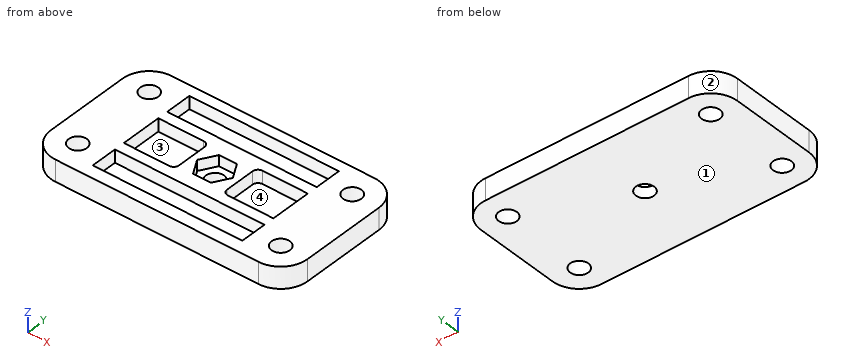
```python
from build123d import *

# Parameters (mm, degrees)
SKETCH1_R           = 1.7
BOSS_EXTRUDE1_DEPTH = 4
CUT_EXTRUDE1_DEPTH  = 2
SKETCH3_W           = 28
SKETCH3_H           = 4.960661027
SKETCH3_W_2         = 9.5
SKETCH3_H_2         = 7.70604726
SKETCH3_H_3         = 4.960661028
CUT_EXTRUDE2_DEPTH  = 2.4
FILLET1_R           = 1


with BuildPart() as part:
    # Sketch1 → Boss-Extrude1 (new body)
    with BuildSketch(Plane.XY):
        with BuildLine():
            Line((-19, -13), (19, -13))
            ThreePointArc((19, -13), (22.535533906, -11.535533906), (24, -8))
            Line((24, -8), (24, 8))
            ThreePointArc((24, 8), (22.535533906, 11.535533906), (19, 13))
            Line((19, 13), (-19, 13))
            ThreePointArc((-19, 13), (-22.535533906, 11.535533906), (-24, 8))
            Line((-24, 8), (-24, -8))
            ThreePointArc((-24, -8), (-22.535533906, -11.535533906), (-19, -13))
        make_face()
        Circle(SKETCH1_R, mode=Mode.SUBTRACT)
        with Locations((19, 8)):
            Circle(SKETCH1_R, mode=Mode.SUBTRACT)
        with Locations((19, -8)):
            Circle(SKETCH1_R, mode=Mode.SUBTRACT)
        with Locations((-19, -8)):
            Circle(SKETCH1_R, mode=Mode.SUBTRACT)
        with Locations((-19, 8)):
            Circle(SKETCH1_R, mode=Mode.SUBTRACT)
    extrude(amount=BOSS_EXTRUDE1_DEPTH)

    # Sketch2 → Cut-Extrude1 (cut)
    with BuildSketch(Plane.XY.offset(4)):
        Polygon((3.348631561, 0), (1.674315781, 2.9), (-1.674315781, 2.9), (-3.348631561, 0), (-1.674315781, -2.9), (1.674315781, -2.9), align=None)
    extrude(amount=-CUT_EXTRUDE1_DEPTH, mode=Mode.SUBTRACT)

    # Sketch3 → Cut-Extrude2 (cut)
    with BuildSketch(Plane.XY.offset(4)):
        with Locations((0, 8.519669486)):
            Rectangle(SKETCH3_W, SKETCH3_H)
        with Locations((-9.25, 0.186315343)):
            Rectangle(SKETCH3_W_2, SKETCH3_H_2)
        with Locations((9.25, 0.186315343)):
            Rectangle(SKETCH3_W_2, SKETCH3_H_2)
        with Locations((0, -8.147038801)):
            Rectangle(SKETCH3_W, SKETCH3_H_3)
    extrude(amount=-CUT_EXTRUDE2_DEPTH, mode=Mode.SUBTRACT)

    # Fillet1
    fillet1_edges = [part.edges().sort_by_distance(p)[0] for p in [
        (-4.5, 4.039338973, 2.8),
        (-4.5, -3.666708287, 2.8),
        (4.5, -3.666708287, 2.8),
        (4.5, 4.039338973, 2.8),
    ]]
    fillet(fillet1_edges, radius=FILLET1_R)


solid = part.part
```
The listing builds one solid part. Answer for the finished solid, in the listing's coordinates (mm). Face numbers are marked on the shaded views. Give positions to 0.01 mm unless a question says otherwise; leave off trailing zeros. Loops run counter-clockwise (first coordinate to the right, second up) from the corner with the lowest first, then second, coordinate; pieces in that order, holes last. Notation, with made-up numbers: (-13, 15.5) - (1, 15.5) arc R15 cw to (1, 34.5) - close; hole circle Ø10 at (23.5, 38.25). An arc over 180 degrees is marked (long way). Answer as CSV lines item,"result". Start each with the question number.
Item 1: A cutting plane is placed at B-B on z = 0.55. Determine the outline of the cut face in (x, y).
Item 2: Each of these flat-tipped pins is pushed along its axis until it touches: pin 1 (4 mm diameter, centred on x = 1, y = -9.5, fed in from +Z); pin 2 (1.5 mm diameter, centred on x = -4, y = -7.5, fed in from +Z). Where does it stop, or does it pass through?
Item 3: A cutting plane is placed at D-D on y = 7.5. Determine the outline of the cut face in (x, z), then the cut area to 3 significant figures.
Item 4: Find the intervals of material crossed by line 1 (Y direction, x = 0.5, z = 2.7); line 2 (Y direction, x = 19, z = 2.55); line 3 (Y direction, x = 10, z = 3.15), in increasing order. Write a range as from..to.
Item 5: A cutting plane is placed at A-A on x = 0. Determine the outline of the cut face in (y, z), then the cut area to 3 significant figures.
Item 6: The mould has two halves that part along X. Classify the marked faces 1, 2, 3 and 4: +X half, -X half, draft (parallel to the pull), parting line (faces both ways), or undercut.
Item 7: A cutting plane is placed at C-C on x = -6.5. Determine the outline of the cut face in (y, z).
Found:
1,outline,"(-24, -8) arc R5 ccw to (-19, -13) - (19, -13) arc R5 ccw to (24, -8) - (24, 8) arc R5 ccw to (19, 13) - (-19, 13) arc R5 ccw to (-24, 8) - close; hole circle Ø3.4 at (-19, -8); hole circle Ø3.4 at (-19, 8); hole circle Ø3.4 at (0, 0); hole circle Ø3.4 at (19, -8); hole circle Ø3.4 at (19, 8)"
2,pin 1,"stops at z = 4"
2,pin 2,"stops at z = 1.6"
3,outline,"(-24, 0) - (-20.62, 0) - (-20.62, 4) - (-24, 4) - close; (-17.38, 0) - (17.38, 0) - (17.38, 4) - (14, 4) - (14, 1.6) - (-14, 1.6) - (-14, 4) - (-17.38, 4) - close; (20.62, 0) - (24, 0) - (24, 4) - (20.62, 4) - close"
3,area,"98.8 mm^2"
4,line 1,"y = -13..-10.63, -5.67..-2.9, 2.9..6.04, 11..13"
4,line 2,"y = -13..-9.7, -6.3..6.3, 9.7..13"
4,line 3,"y = -13..-10.63, -5.67..-3.67, 4.04..6.04, 11..13"
5,outline,"(-13, 0) - (-1.7, 0) - (-1.7, 2) - (-2.9, 2) - (-2.9, 4) - (-5.67, 4) - (-5.67, 1.6) - (-10.63, 1.6) - (-10.63, 4) - (-13, 4) - close; (1.7, 0) - (13, 0) - (13, 4) - (11, 4) - (11, 1.6) - (6.04, 1.6) - (6.04, 4) - (2.9, 4) - (2.9, 2) - (1.7, 2) - close"
5,area,"61.8 mm^2"
6,face 1,"draft"
6,face 2,"-X half"
6,face 3,"undercut"
6,face 4,"undercut"
7,outline,"(-13, 0) - (13, 0) - (13, 4) - (11, 4) - (11, 1.6) - (6.04, 1.6) - (6.04, 4) - (4.04, 4) - (4.04, 1.6) - (-3.67, 1.6) - (-3.67, 4) - (-5.67, 4) - (-5.67, 1.6) - (-10.63, 1.6) - (-10.63, 4) - (-13, 4) - close"
